Source: CAD feature listing. Evaluate the final solid. Frame: model axes, mm. A direction names the side the tool comes from. Give positions to 0.01 mm unless a question says otherwise; leave off trailing zeros. Order: outer loops, then holes, each group sorted by start corner. A loop starts at its lowest first (then second) coordinate and runs counter-clockwise, first axis right, second up. Notation, with made-up numbers: M 39.5,-31.75 L 75.5,-31.75 A24 cw 75.5,-8.75 Z; hole C 56,-8.75 d5. An arc over 180 degrees is marked long. Use CSV: the item, a comma, the result in double quotes. Start each with the question number.
1. Reachability of faces 1 (the flat face through (-104.25, -17, 2)), 2 (the flat face through (-78.85, -10, 2)) from +Z, -Z, +X, -X, +Y, -Y: full face, straight path, thin tool, end or side. Return the list, or none.
2. Section query B-B, the plane x = -109.75. Return the cut outline in (y, z) (1 decimal), plus the area to 3 significant figures.
3. Section query D-D, the plane x = -97.75. Return the cut outline in (y, z) (1 decimal).
4. Line query: line 1 along X through (y, z) = (-21.5, 2.05); line 2 along X through (y, z) = (-10, 3.05); line 3 along Y through (x, z) = (-93, 3). Output: solid intervals per line, ascending. Write a range as [from, to].
5. Pin query (flat end, axial travel): P1, Ø3.5, axis at x = -85.75, y = -9.76, coming from the +Z side. Return the tip coordinate at first contact, or that it passes through.
6. Section query C-C, the plane y = -4.5. Return the cut outline in (x, z) (3 decimals), plus the area to 3 significant figures.
7. Section query A-A, the plane z = 1.25. Return the cut outline in (x, y), plus the area to 3 significant figures.
8. Mould query, pull axis X, two halves, no side actions, for faces 3 (the flat face through (-116.65, -10, 2)), 4 (the flat face through (-85, -24.762, 2)), 5 (the cylindrical face through (-107.6, -9.1, 1.6)). Classes: released by +X, released by -X, zero draft, split by the parting line, or undercut.
from build123d import *

# Parameters (mm, degrees)
SKETCH1_W            = 299.7
SKETCH1_H            = 76.075
BOSS_EXTRUDE1_DEPTH  = 3.175
CUT_EXTRUDE4_DEPTH   = 155.634907221
SKETCH3_R            = 6.5
CUT_EXTRUDE5_DEPTH   = 155.634907221
M4_CLEARANCE_HOLE1_D = 4.5
SKETCH12_W           = 144
SKETCH12_H           = 3.175
BOSS_EXTRUDE2_DEPTH  = 6.35
SKETCH14_R           = 2.25
SKETCH14_W           = 12.4
SKETCH14_H           = 13.275
CUT_EXTRUDE7_DEPTH   = 157.318115653


with BuildPart() as part:
    # Sketch1 → Boss-Extrude1 (new body)
    with BuildSketch(Plane.XY):
        Rectangle(SKETCH1_W, SKETCH1_H)
    extrude(amount=BOSS_EXTRUDE1_DEPTH)

    # Sketch8 → Cut-Extrude4 (cut, through all)
    with BuildSketch(Plane.XY.offset(3.175)):
        with BuildLine():
            Line((121.65, 18.5125), (123.65, 18.5125))
            ThreePointArc((123.65, 18.5125), (127.185533906, 17.048033906), (128.65, 13.5125))
            Line((128.65, 13.5125), (128.65, -27.282435401))
            ThreePointArc((128.65, -27.282435401), (127.185533906, -30.817969307), (123.65, -32.282435401))
            Line((123.65, -32.282435401), (121.65, -32.282435401))
            ThreePointArc((121.65, -32.282435401), (118.114466094, -30.817969307), (116.65, -27.282435401))
            Line((116.65, -27.282435401), (116.65, 13.5125))
            ThreePointArc((116.65, 13.5125), (118.114466094, 17.048033906), (121.65, 18.5125))
        make_face()
        with BuildLine():
            Line((128.65, -38.0375), (128.65, -27.282435401))
            ThreePointArc((128.65, -27.282435401), (127.185533906, -30.817969307), (123.65, -32.282435401))
            Line((123.65, -32.282435401), (121.65, -32.282435401))
            ThreePointArc((121.65, -32.282435401), (118.114466094, -30.817969307), (116.65, -27.282435401))
            Line((116.65, -27.282435401), (116.65, -38.0375))
            Line((116.65, -38.0375), (128.65, -38.0375))
        make_face()
    cut_extrude4 = extrude(amount=-CUT_EXTRUDE4_DEPTH, mode=Mode.SUBTRACT)

    # Mirror3: Cut-Extrude4 across plane
    add(cut_extrude4.mirror(Plane(origin=(0, 0, 0), x_dir=(0, 0, 1), z_dir=(1, 0, 0))), mode=Mode.SUBTRACT)

    # Sketch3 → Cut-Extrude5 (cut, through all)
    with BuildSketch(Plane(origin=(0, 0, 0), x_dir=(-1, 0, 0), z_dir=(0, 0, -1))):
        with Locations((-97.75, -9.7625)):
            Circle(SKETCH3_R)
        with BuildLine():
            Line((-104.25, -38.0375), (-91.25, -38.0375))
            Line((-91.25, -38.0375), (-91.25, -9.7625))
            ThreePointArc((-91.25, -9.7625), (-97.75, -16.2625), (-104.25, -9.7625))
            Line((-104.25, -9.7625), (-104.25, -38.0375))
        make_face()
        with Locations((97.75, -9.7625)):
            Circle(SKETCH3_R)
        with BuildLine():
            Line((91.25, -38.0375), (104.25, -38.0375))
            Line((104.25, -38.0375), (104.25, -9.7625))
            ThreePointArc((104.25, -9.7625), (97.75, -16.2625), (91.25, -9.7625))
            Line((91.25, -9.7625), (91.25, -38.0375))
        make_face()
    extrude(amount=-CUT_EXTRUDE5_DEPTH, mode=Mode.SUBTRACT)

    # M4 Clearance Hole1 (through all)
    with Locations(Plane(origin=(0, 0, 0), x_dir=(-1, 0, 0), z_dir=(0, 0, -1))):
        with Locations((-85.75, -9.7625), (-109.75, -9.7625), (109.75, -9.7625), (85.75, -9.7625)):
            Hole(M4_CLEARANCE_HOLE1_D / 2)

    # Sketch12 → Boss-Extrude2 (add)
    with BuildSketch(Plane.XZ.offset(38.0375)):
        with Locations((0, 1.5875)):
            Rectangle(SKETCH12_W, SKETCH12_H)
    extrude(amount=BOSS_EXTRUDE2_DEPTH)

    # Sketch14 → Cut-Extrude7 (cut, through all)
    # profile 1 of 2: a face of its own
    with BuildSketch(Plane.XY.offset(3.175)):
        with BuildLine():
            Line((-78.85, -24.7625), (-91.25, -24.7625))
            Line((-91.25, -24.7625), (-91.25, -38.0375))
            Line((-91.25, -38.0375), (-72, -38.0375))
            Line((-72, -38.0375), (-72, -44.3875))
            Line((-72, -44.3875), (72, -44.3875))
            Line((72, -44.3875), (72, -38.0375))
            Line((72, -38.0375), (91.25, -38.0375))
            Line((91.25, -38.0375), (91.25, -9.7625))
            ThreePointArc((91.25, -9.7625), (97.75, -3.2625), (104.25, -9.7625))
            Line((104.25, -9.7625), (104.25, -38.0375))
            Line((104.25, -38.0375), (116.65, -38.0375))
            Line((116.65, -38.0375), (116.65, 13.5125))
            ThreePointArc((116.65, 13.5125), (118.114466094, 17.048033906), (121.65, 18.5125))
            Line((121.65, 18.5125), (123.65, 18.5125))
            ThreePointArc((123.65, 18.5125), (127.185533906, 17.048033906), (128.65, 13.5125))
            Line((128.65, 13.5125), (128.65, -38.0375))
            Line((128.65, -38.0375), (149.85, -38.0375))
            Line((149.85, -38.0375), (149.85, 38.0375))
            Line((149.85, 38.0375), (-149.85, 38.0375))
            Line((-149.85, 38.0375), (-149.85, -38.0375))
            Line((-149.85, -38.0375), (-128.65, -38.0375))
            Line((-128.65, -38.0375), (-128.65, 13.5125))
            ThreePointArc((-128.65, 13.5125), (-127.185533906, 17.048033906), (-123.65, 18.5125))
            Line((-123.65, 18.5125), (-121.65, 18.5125))
            ThreePointArc((-121.65, 18.5125), (-118.114466094, 17.048033906), (-116.65, 13.5125))
            Line((-116.65, 13.5125), (-116.65, 5.2375))
            Line((-116.65, 5.2375), (-78.85, 5.2375))
            Line((-78.85, 5.2375), (-78.85, -24.7625))
        make_face()
        with Locations((85.75, -9.7625)):
            Circle(SKETCH14_R, mode=Mode.SUBTRACT)
        with Locations((109.75, -9.7625)):
            Circle(SKETCH14_R, mode=Mode.SUBTRACT)
    # profile 2 of 2: a face of its own
    with BuildSketch(Plane.XY.offset(3.175)):
        with Locations((-110.45, -31.4)):
            Rectangle(SKETCH14_W, SKETCH14_H)
    extrude(amount=-CUT_EXTRUDE7_DEPTH, mode=Mode.SUBTRACT)


solid = part.part
Result set:
1,face 1,"+Z, -Z, -Y"
1,face 2,"+Z, -Z, +X, +Y, -Y"
2,outline,"M -24.8,0 L -12,0 L -12,3.2 L -24.8,3.2 Z; M -7.5,0 L 5.2,0 L 5.2,3.2 L -7.5,3.2 Z"
2,area,"81.0 mm2"
3,outline,"M -3.3,0 L 5.2,0 L 5.2,3.2 L -3.3,3.2 Z"
4,line 1,"[-116.65, -104.25], [-91.25, -78.85]"
4,line 2,"[-116.65, -111.99], [-107.51, -104.25], [-91.25, -87.99], [-83.51, -78.85]"
4,line 3,"[-5.33, 5.24]"
5,P1,"through"
6,outline,"M -116.65,0 L -101.565,0 L -101.565,3.175 L -116.65,3.175 Z; M -93.935,0 L -78.85,0 L -78.85,3.175 L -93.935,3.175 Z"
6,area,"95.8 mm2"
7,outline,"M -116.65,-24.76 L -104.25,-24.76 L -104.25,-9.76 A6.5 cw -91.25,-9.76 L -91.25,-24.76 L -78.85,-24.76 L -78.85,5.24 L -116.65,5.24 Z; hole C -109.75,-9.76 d4.5; hole C -85.75,-9.76 d4.5"
7,area,"841 mm2"
8,face 3,"released by -X"
8,face 4,"zero draft"
8,face 5,"undercut"
